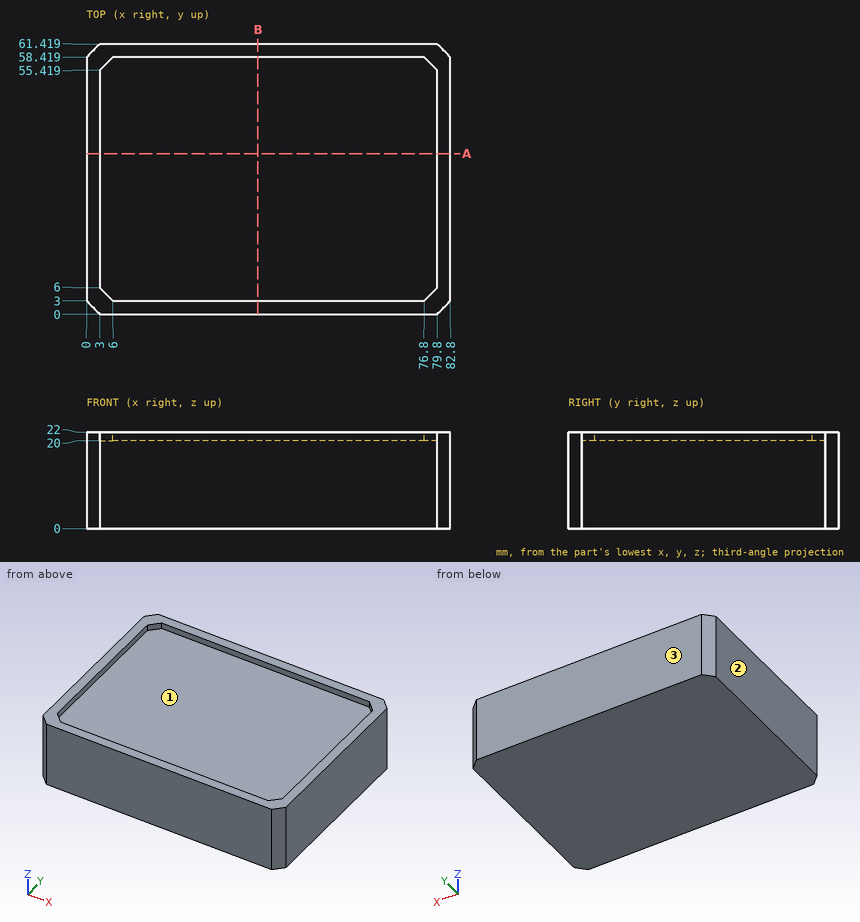
Source: three-view drawing plus pictorial views. Frame: mm from the lowest corner of the part. Coordinates: 2 decimals unless noted, no trailing zeros. Loops run counter-clockwise (first coordinate to the right, second up) from the corner with the lowest first, then second, coordinate; pieces in that order, holes last. Notation, with made-up numbers: (20.25, -14.75) - (37.25, -14.75) arc R17 cw to (37.25, 5.25) - close; hole circle Ø11 at (52.25, 89.5). An arc over 180 degrees is marked (long way). One line per item, written item: value. Start each with the question number.
1. Ray query, L1, parallel to X at y = 51, z = 21; L2, parallel to Z at x = 19, y = 45. Return the intervals inside material, ascending.
2. Section A-A (y = 36.5). Return the cut outline in (x, z).
3. Section B-B (x = 39). Return the cut outline in (y, z), and give its area (3 significant figures).
4. Mould query, pull axis Y, two halves, no side actions, for the marked faces 1, 2 and 3. Classes: pulls with the +Y half, pulls with the -Y half, needs draft (parallel to the pull), parting line crosses it, or undercut.
5. Contact query for flat-ended pins moving along their axis: P1, Ø2, axis at x = 42.5, z = 18.5, coming from the -Y side; P2, Ø3, axis at x = 68.5, y = 10, coming from the +Z side. Output: stop coordinate, or through.
Verdict:
1. L1: x = 0 to 3, 79.8 to 82.8
1. L2: z = 0 to 20
2. outline: (0, 0) - (82.8, 0) - (82.8, 22) - (79.8, 22) - (79.8, 20) - (3, 20) - (3, 22) - (0, 22) - close
3. outline: (0, 0) - (61.42, 0) - (61.42, 22) - (58.42, 22) - (58.42, 20) - (3, 20) - (3, 22) - (0, 22) - close
3. area: 1,240 mm2
4. face 1: undercut
4. face 2: needs draft
4. face 3: pulls with the +Y half
5. P1: stops at y = 0
5. P2: stops at z = 20
